```python
from build123d import *

# Parameters (mm, degrees)
ESBO_O1_W                = 7
ESBO_O1_H                = 11
RESSALTO_EXTRUS_O1_DEPTH = 2
ESBO_O2_W                = 7
ESBO_O2_H                = 2
RESSALTO_EXTRUS_O2_DEPTH = 3.5
ESBO_O3_W                = 7
ESBO_O3_H                = 2
RESSALTO_EXTRUS_O3_DEPTH = 1.5
ESBO_O4_R                = 1.55
CORTE_EXTRUS_O1_DEPTH    = 2
FILETE1_R                = 0.5


with BuildPart() as part:
    # Esboço1 → Ressalto-extrusão1 (new body)
    with BuildSketch(Plane(origin=(0, 0, 0), x_dir=(1, 0, 0), z_dir=(0, 1, 0))):
        Rectangle(ESBO_O1_W, ESBO_O1_H)
    extrude(amount=RESSALTO_EXTRUS_O1_DEPTH)

    # Esboço2 → Ressalto-extrusão2 (add)
    with BuildSketch(Plane(origin=(0, 2, 0), x_dir=(1, 0, 0), z_dir=(0, 1, 0))):
        with Locations((0, 4.5)):
            Rectangle(ESBO_O2_W, ESBO_O2_H)
    extrude(amount=RESSALTO_EXTRUS_O2_DEPTH)

    # Esboço3 → Ressalto-extrusão3 (add)
    with BuildSketch(Plane(origin=(0, 0, -5.5), x_dir=(-1, 0, 0), z_dir=(0, 0, -1))):
        with Locations((0, 4.5)):
            Rectangle(ESBO_O3_W, ESBO_O3_H)
    extrude(amount=RESSALTO_EXTRUS_O3_DEPTH)

    # Esboço4 → Corte-extrusão1 (cut)
    with BuildSketch(Plane(origin=(0, 2, 0), x_dir=(1, 0, 0), z_dir=(0, 1, 0))):
        with Locations(Location((0, -1, 0), (0, 0, 270))):
            Circle(ESBO_O4_R)
    extrude(amount=-CORTE_EXTRUS_O1_DEPTH, mode=Mode.SUBTRACT)

    # Filete1
    filete1_edges = [part.edges().sort_by_distance(p)[0] for p in [
        (-3.5, 2, 1),
        (0, 2, -3.5),
        (-3.5, 3.75, -3.5),
        (0, 2, 5.5),
        (3.5, 3.75, -3.5),
        (-3.5, 5.5, -5.25),
        (0, 5.5, -3.5),
        (3.5, 5.5, -5.25),
        (0, 5.5, -7),
        (3.5, 2, 1),
        (3.5, 1, 5.5),
        (-3.5, 1, 5.5),
    ]]
    fillet(filete1_edges, radius=FILETE1_R)


solid = part.part
```
Work out the finished part from the listing and answer in its coordinate system (mm). A direction names the side the tool comes from. Round coordinates to 2 decimals unless told otherwise and drop trailing zeros. Loops run counter-clockwise (first coordinate to the right, second up) from the corner with the lowest first, then second, coordinate; pieces in that order, holes last. Notation, with made-up numbers: M 4.25,-24 L 11.25,-24 A18 ccw 11.25,-9 Z; hole C 68.5,77 d1. An arc over 180 degrees is marked long. Use CSV: the item, a comma, the result in double quotes.
Q1. Section A-A, the plane y = 0.5 is taken. Determine the outline of the cut face in (x, z).
Determined:
outline,"M -3.5,-5.5 L 3.5,-5.5 L 3.5,5 A0.5 ccw 3,5.5 L -3,5.5 A0.5 ccw -3.5,5 Z; hole C 0,1 d3.1"
Q2. Each of these flat-tipped pins is pushed along its axis until it touches: pin 1 (2 mm diameter, centred on x = -1, y = 3.5, fed in from +Z); pin 2 (4 mm diameter, centred on x = -1, z = -0.5, fed in from +Y); pin 3 (1.9 mm diameter, centred on x = 0, z = 1, fed in from -Y); pin 4 (0.8 mm diameter, centred on x = -0.5, z = -6, fed in from -Y). Where does it stop, or does it pass through?
Determined:
pin 1,"z = -3.5"
pin 2,"y = 2"
pin 3,"through"
pin 4,"y = 3.5"
Q3. Section C-C, the plane x = 0 is taken. Determine the outline of the cut face in (y, z).
Determined:
outline,"M 0,-5.5 L 3.5,-5.5 L 3.5,-7 L 5,-7 A0.5 ccw 5.5,-6.5 L 5.5,-4 A0.5 ccw 5,-3.5 L 2.5,-3.5 A0.5 cw 2,-3 L 2,-0.55 L 0,-0.55 Z; M 0,2.55 L 2,2.55 L 2,5 A0.5 ccw 1.5,5.5 L 0,5.5 Z"
Q4. The mould has two halves that part along X. Classify faces 4 (the cylindrical face through (0.466, 1.014, 2.478)), 5 (the flat face through (0, 1, 5.5)), 6 (the flat face through (-3.5, 1, -2)): pulls with the +X half, pulls with the -X half, needs draft (parallel to the pull), parting line crosses it, or undercut.
Determined:
face 4,"undercut"
face 5,"needs draft"
face 6,"pulls with the -X half"
Q5. Consider L1, parallel to X at y = 1.55, z = 1; L2, parallel to Z at x = 3, y = 2.5; L3, parallel to Y at x = -1.5, z = 4.75. Determine where each line is inside the solid, lowest interval first.
Determined:
L1,"-3.5 to -1.55, 1.55 to 3.5"
L2,"-5.5 to -3.5"
L3,"0 to 2"
Q6. A tool of negligible diameter and unlimited length cuts with its end or side. For faces 1 (the flat face through (0, 2, -5.5)), 2 (the flat face through (3.5, 1, -2)), 3 (the flat face through (0, 2, -1)), from which of +Z, -Z, +X, -X, +Y, -Y can it reach the whole face along a straight path? Write none if from no direction.
Determined:
face 1,"-Z, +X, -X, -Y"
face 2,"+Z, -Z, +X, +Y, -Y"
face 3,"+Z, +X, -X, +Y"
Q7. Section D-D, the plane y = 4.35 is taken. Determine the outline of the cut face in (x, z).
Determined:
outline,"M -3.5,-7 L 3.5,-7 L 3.5,-4 A0.5 ccw 3,-3.5 L -3,-3.5 A0.5 ccw -3.5,-4 Z"
Q8. Section B-B, the plane z = 1 is taken. Determine the outline of the cut face in (x, y), then the cut area to 3 significant figures.
Determined:
outline,"M -3.5,0 L -1.55,0 L -1.55,2 L -3,2 A0.5 ccw -3.5,1.5 Z; M 1.55,0 L 3.5,0 L 3.5,1.5 A0.5 ccw 3,2 L 1.55,2 Z"
area,"7.69 mm2"
